from build123d import *

# Parameters (mm, degrees)
SKETCH_W     = 28
SKETCH_H     = 40
PAD_DEPTH    = 7
SKETCH001_W  = 5
SKETCH001_H  = 40
PAD001_DEPTH = 5
SKETCH002_W  = 5
SKETCH002_H  = 5
PAD002_DEPTH = 33.5
SKETCH003_W  = 3
SKETCH003_H  = 5
PAD003_DEPTH = 5
SKETCH004_W  = 4
SKETCH004_H  = 5
PAD004_DEPTH = 4
SKETCH005_W  = 12
SKETCH005_H  = 10
POCKET_DEPTH = 9.001
FILLET_R     = 6.5
CHAMFER_SIZE = 3


with BuildPart() as part:
    # Sketch → Pad (new body)
    with BuildSketch(Plane.XY):
        with Locations((14, 20)):
            Rectangle(SKETCH_W, SKETCH_H)
    extrude(amount=PAD_DEPTH)

    # Sketch001 (on Face6 of Pad) → Pad001 (join)
    with BuildSketch(Plane.XY.offset(7)):
        with Locations((2.5, 20)):
            Rectangle(SKETCH001_W, SKETCH001_H)
    extrude(amount=PAD001_DEPTH)

    # Sketch002 (on Face7 of Pad001) → Pad002 (join)
    with BuildSketch(Plane(origin=(0, 0, 0), x_dir=(0, -1, 0), z_dir=(-1, 0, 0))):
        with Locations((-37.5, 9.5)):
            Rectangle(SKETCH002_W, SKETCH002_H)
        with Locations((-2.5, 9.5)):
            Rectangle(SKETCH002_W, SKETCH002_H)
    extrude(amount=PAD002_DEPTH)

    # Sketch003 (on Face9 of Pad002) → Pad003 (join)
    with BuildSketch(Plane(origin=(0, 0, 7), x_dir=(1, 0, 0), z_dir=(0, 0, -1))):
        with Locations((-32, -2.5)):
            Rectangle(SKETCH003_W, SKETCH003_H)
        with Locations((-32, -37.5)):
            Rectangle(SKETCH003_W, SKETCH003_H)
    extrude(amount=PAD003_DEPTH)

    # Sketch004 (on Face10 of Pad003) → Pad004 (join)
    with BuildSketch(Plane(origin=(0, 0, 2), x_dir=(1, 0, 0), z_dir=(0, 0, -1))):
        with Locations((-31.5, -2.5)):
            Rectangle(SKETCH004_W, SKETCH004_H)
        with Locations((-31.5, -37.5)):
            Rectangle(SKETCH004_W, SKETCH004_H)
    extrude(amount=PAD004_DEPTH)

    # Sketch005 (on Face3 of Pad004) → Pocket (cut, through all)
    with BuildSketch(Plane.XY.offset(7)):
        with Locations((22, 20)):
            Rectangle(SKETCH005_W, SKETCH005_H)
    extrude(amount=-POCKET_DEPTH, mode=Mode.SUBTRACT)

    # Fillet
    fillet_edges = [part.edges().sort_by_distance(p)[0] for p in [
        (28, 7.5, 7),
        (28, 32.5, 7),
    ]]
    fillet(fillet_edges, radius=FILLET_R)

    # Chamfer
    chamfer_edges = [part.edges().sort_by_distance(p)[0] for p in [
        (-29.5, 37.5, -2),
        (-29.5, 2.5, -2),
    ]]
    chamfer(chamfer_edges, length=CHAMFER_SIZE)


solid = part.part
Build history of the part. All positions in model axes, mm. A direction names the side the tool comes from. Round coordinates to 2 decimals unless told otherwise and drop trailing zeros. Write each loop counter-clockwise with the first axis right and the second up, starting at its lowest first coordinate (ties: lowest second). Pieces come first, ordered by that corner, then holes. Notation, with made-up numbers: M 32,-1 L 66,-1 A32 cw 66,29 Z; hole C 79.5,-13 d10. An arc over 180 degrees is marked long. Use CSV: the item, a comma, the result in double quotes.
1. Tool access for faces 4 (the face through (16, 20, 4)), 5 (the face through (5, 20, 9)), 6 (the face through (-30.5, 3, 5)), 7 (the face through (-31, 37.5, -0.5)), 8 (the face through (-20, 35, 8)): list every direction of +Z, -Z, +X, -X, +Y, -Y with a clear straight run to the whole face (end or side of a thin tool).
Reply:
face 4,"+Z, -Z, +X"
face 5,"+Z, +X, +Y, -Y"
face 6,"+Y, -Y"
face 7,"-Z, +Y, -Y"
face 8,"+Z, -Z, -X"
2. Saw through at A-A (x = 18.5). Give the cut face in (y, z).
Reply:
outline,"M 0,0 L 15,0 L 15,7 L 0,7 Z; M 25,0 L 40,0 L 40,7 L 25,7 Z"
3. Saw through at D-D (y = 16). Give the cut face in (x, z).
Reply:
outline,"M 0,0 L 16,0 L 16,7 L 5,7 L 5,12 L 0,12 Z"
4. Flat gauge pins, fed straight in: pin 1 (2 mm diameter, centred on y = 23.5, z = 1.5, fed in from -X); pin 2 (8 mm diameter, centred on y = 20, z = 3, fed in from +X); pin 3 (1.5 mm diameter, centred on x = -15.5, y = 1.5, fed in from -Z). Where does each tip first touch, or does it go through?
Reply:
pin 1,"stops at x = 0"
pin 2,"stops at x = 16"
pin 3,"stops at z = 7"
5. Wall check: probe 1 along Y at (x, z) = (-8.5, 8.75); probe 2 along X at (y, z) = (22, 6.5); probe 3 along Z at (x, y) = (-26, 38.5). Give the ranges that are in metal, low to high. Write a range as from..to.
Reply:
probe 1,"y = 0..5, 35..40"
probe 2,"x = 0..16"
probe 3,"z = 7..12"
6. Saw through at B-B (z = 3). Give the cut face in (x, y), plus the area to 4 significant figures.
Reply:
outline,"M -33.5,0 L -30.5,0 L -30.5,5 L -33.5,5 Z; M -33.5,35 L -30.5,35 L -30.5,40 L -33.5,40 Z; M 0,0 L 27.5,0 L 27.5,15 L 16,15 L 16,25 L 27.5,25 L 27.5,40 L 0,40 Z"
area,"1,015 mm²"
7. Saw through at C-C (z = 9). Give the cut face in (x, y), plus the area to 3 significant figures.
Reply:
outline,"M -33.5,0 L 5,0 L 5,40 L -33.5,40 L -33.5,35 L 0,35 L 0,5 L -33.5,5 Z"
area,"535 mm²"
8. Two-plate mould, pull along Y, no slides. Class faces 1 (the face through (14, 20, 0)), 2 (the face through (-3, 0, 8)), 3 (the face through (22, 25, 4)): +Y half, -Y half, draft (parallel to the pull), parting line (faces both ways), or undercut.
Reply:
face 1,"draft"
face 2,"-Y half"
face 3,"undercut"
